Check sheet for the drawn part. Datum: minimum x, y, z corner. Units: mm. A direction names the side the tool comes from. Give positions to 0.01 mm unless a question says otherwise; leave off trailing zeros. Write each loop counter-clockwise with the first axis right and the second up, starting at its lowest first coordinate (ties: lowest second). Pieces come first, ordered by that corner, then holes.
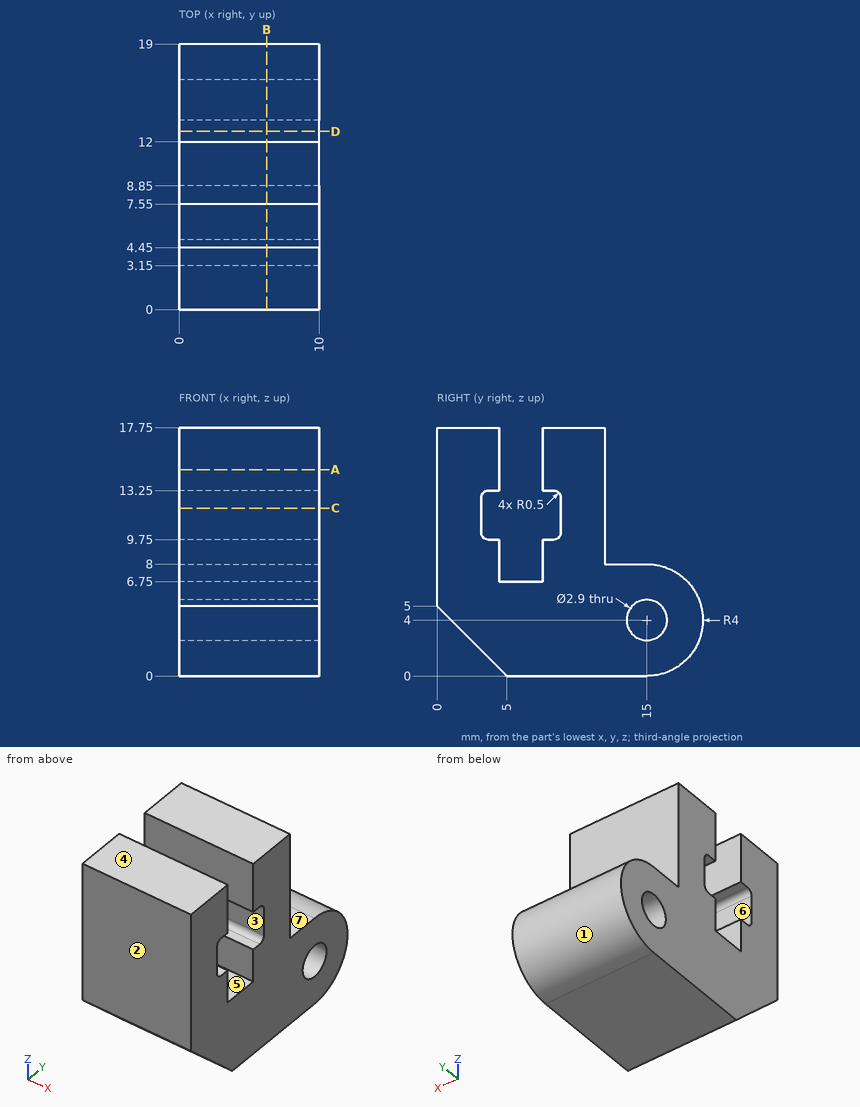
1) Access from +Z, -Z, +X, -X, +Y, -Y to the whole of each face (thin tool, end or side, straight path). Record for the marked faces 4, 5, 6 and 7.
2) Sectioned sample at C-C on z = 12. Record the boundary of the cut face in (x, y).
3) Scan lines: L1, parallel to Y at x = 1.75, z = 12.5; L2, parallel to Z at x = 5, y = 13.5; L3, parallel to Y at x = 4.25, z = 16.25. Record each from-to range of solid material in increasing order.
4) Sectioned sample at B-B on x = 6.25. Record the boundary of the cut face in (y, z).
5) Gauge pin test, flat ends, axial feed: pin 1 (3 mm diameter, centred on x = 5, z = 11, fed in from +Y); pin 2 (2.5 mm diameter, centred on x = 7.5, y = 14, fed in from +Z); pin 3 (0.9 mm diameter, centred on x = 6, y = 5.5, fed in from +Z). Record the tip position at first contact, or that the pin passes through.
6) Sectioned sample at D-D on y = 12.75. Record the boundary of the cut face in (x, z), then the cut area to 3 significant figures.
7) Draft check along Y on the marked faces 1, 2 and 3. Enter one of: +Y half, -Y half, draft (parallel to the pull), parting line (faces both ways), or undercut.
8) Sectioned sample at A-A on z = 14.75. Record the boundary of the cut face in (x, y).
Answers below:
1. face 4: +Z, +X, -X, +Y, -Y
1. face 5: +Z, +X, -X
1. face 6: +X, -X
1. face 7: +Z, +X, -X, +Y
2. outline: (0, 0) - (10, 0) - (10, 3.15) - (0, 3.15) - close; (0, 8.85) - (10, 8.85) - (10, 12) - (0, 12) - close
3. L1: y = 0 to 3.15, 8.85 to 12
3. L2: z = 0 to 8
3. L3: y = 0 to 4.45, 7.55 to 12
4. outline: (0, 5) - (5, 0) - (15, 0) arc R4 ccw to (15, 8) - (12, 8) - (12, 17.75) - (7.55, 17.75) - (7.55, 13.25) - (8.35, 13.25) arc R0.5 cw to (8.85, 12.75) - (8.85, 10.25) arc R0.5 cw to (8.35, 9.75) - (7.55, 9.75) - (7.55, 6.75) - (4.45, 6.75) - (4.45, 9.75) - (3.65, 9.75) arc R0.5 cw to (3.15, 10.25) - (3.15, 12.75) arc R0.5 cw to (3.65, 13.25) - (4.45, 13.25) - (4.45, 17.75) - (0, 17.75) - close; hole circle Ø2.9 at (15, 4)
5. pin 1: stops at y = 12
5. pin 2: stops at z = 8
5. pin 3: stops at z = 6.75
6. outline: (0, 0) - (10, 0) - (10, 8) - (0, 8) - close
6. area: 80.0 mm2
7. face 1: +Y half
7. face 2: -Y half
7. face 3: undercut
8. outline: (0, 0) - (10, 0) - (10, 4.45) - (0, 4.45) - close; (0, 7.55) - (10, 7.55) - (10, 12) - (0, 12) - close
